from build123d import *

# Parameters (mm, degrees)
SKETCH_1_W          = 60
SKETCH_1_H          = 18
SKETCH_1_W_2        = 22.5
SKETCH_1_H_2        = 12
EXTRUDE_1_DEPTH     = 21
SKETCH_2_W          = 60
SKETCH_2_H          = 18
EXTRUDE_2_DEPTH     = 3
SKETCH_3_W          = 6
SKETCH_3_H          = 3
CUT_EXTRUDE_1_DEPTH = 6
SKETCH_4_R          = 2.75
EXTRUDE_3_DEPTH     = 5
SKETCH_6_R          = 1
CUT_EXTRUDE_2_DEPTH = 5
FILLET_1_R          = 1


with BuildPart() as part:
    # 草图1 → 凸台-拉伸1 (new body)
    with BuildSketch(Plane(origin=(0, 0, 0), x_dir=(1, 0, 0), z_dir=(0, 1, 0))):
        Rectangle(SKETCH_1_W, SKETCH_1_H)
        with Locations((-12.75, 0)):
            Rectangle(SKETCH_1_W_2, SKETCH_1_H_2, mode=Mode.SUBTRACT)
    extrude(amount=EXTRUDE_1_DEPTH)

    # 草图2 → 凸台-拉伸2 (add)
    with BuildSketch(Plane.XZ):
        Rectangle(SKETCH_2_W, SKETCH_2_H)
    extrude(amount=EXTRUDE_2_DEPTH)

    # 草图3 → 切除-拉伸1 (cut)
    with BuildSketch(Plane.ZY.offset(30)):
        with Locations((0, 1.5)):
            Rectangle(SKETCH_3_W, SKETCH_3_H)
    extrude(amount=-CUT_EXTRUDE_1_DEPTH, mode=Mode.SUBTRACT)

    # 草图4 → 凸台-拉伸3 (add)
    with BuildSketch(Plane.XZ.offset(3)):
        with Locations(Location((-18, 0, 0), (0, 0, 270))):
            Circle(SKETCH_4_R)
    extrude(amount=EXTRUDE_3_DEPTH)

    # 草图6 → 切除-拉伸2 (cut)
    with BuildSketch(Plane(origin=(0, 21, 0), x_dir=(1, 0, 0), z_dir=(0, 1, 0))):
        with Locations(Location((-26.75, 0, 0), (0, 0, 270))):
            Circle(SKETCH_6_R)
        with Locations(Location((1.25, 0, 0), (0, 0, 270))):
            Circle(SKETCH_6_R)
    extrude(amount=-CUT_EXTRUDE_2_DEPTH, mode=Mode.SUBTRACT)

    # 圆角1
    fillet_1_edges = [part.edges().sort_by_distance(p)[0] for p in [
        (-30, 21, 0),
        (0, 21, 9),
        (-30, -3, 0),
        (0, -3, -9),
        (30, -3, 0),
        (0, -3, 9),
        (30, 21, 0),
        (-30, 1.5, -3),
        (-30, 0, 0),
        (-30, 1.5, 3),
        (-30, 3, 0),
        (-18, -3, 2.75),
        (0, 21, -9),
        (30, 9, 9),
        (-30, 9, 9),
        (-30, 9, -9),
        (30, 9, -9),
    ]]
    fillet(fillet_1_edges, radius=FILLET_1_R)


solid = part.part
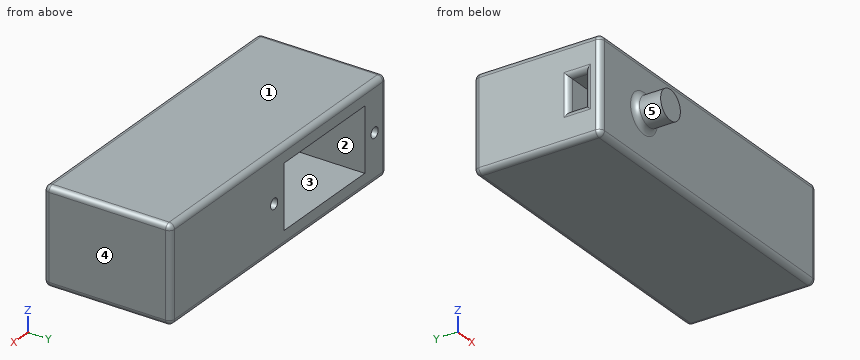
Part model, mm, in its own coordinate system. Face numbers are marked on the shaded views. A direction names the side the tool comes from. Coordinates: 2 decimals unless noted, no trailing zeros. Order: outer loops, then holes, each group sorted by start corner. A loop starts at its lowest first (then second) coordinate and runs counter-clockwise, first axis right, second up. Notation, with made-up numbers: M 44,21 L 77,21 A11 ccw 77,31 Z; hole C 70.25,41 d10. An arc over 180 degrees is marked long. One line per question, with ' | ' between items.
Q1. Slice it at D-D (x = 1.25). Give the cut face in (y, z), and give its area (3 significant figures).
A:
outline: M -3,-8 A1 ccw -2,-9 L 20,-9 A1 ccw 21,-8 L 21,-1 L 16,-1 L 16,1 L 21,1 L 21,8 A1 ccw 20,9 L -2,9 A1 ccw -3,8 Z | area: 421 mm^2
Q2. Drill centre lines: line 1 (X direction, y = 19.85, z = 0); line 2 (X direction, y = 17, z = 4.25); line 3 (Z direction, x = -2.5, y = 11.5). Where is each one in solid material? Low to high.
A:
line 1: x = -30 to -27.75, -25.75 to -24, -1.5 to 0.25, 2.25 to 30 | line 2: x = -30 to -24, -1.5 to 30 | line 3: z = -9 to -6, 6 to 9
Q3. Pin check, flat tips, straight feed: P1, Ø1.6, axis at x = 1, z = -0.5, coming from the +Y side; P2, Ø3.5, axis at x = -16, z = 0.5, coming from the +Y side; P3, Ø1.5, axis at x = -27, z = 0.5, coming from the -Y side; P4, Ø1.6, axis at x = 1.25, z = 0, coming from the +Y side. Stop position of each tip, or through.
A:
P1: stops at y = 21 | P2: stops at y = 0 | P3: stops at y = -3 | P4: stops at y = 16
Q4. 3-axis set-ups, long thin cutter, end or side, ignore diameter. For the marked faces 1 and 2: which of +Z, -Z, +X, -X, +Y, -Y reach the whole face in a straight line?
A:
face 1: +Z, +X, -X, +Y, -Y | face 2: +Y
Q5. Two-plate mould, pull along Z, no slides. Class the marked faces 3, 4 and 5: +Z half, -Z half, draft (parallel to the pull), parting line (faces both ways), or undercut.
A:
face 3: undercut | face 4: draft | face 5: parting line
Q6. Slice it at B-B (y = 19). Give the cut face in (x, z).
A:
outline: M -30,-8 A1 ccw -29,-9 L 29,-9 A1 ccw 30,-8 L 30,8 A1 ccw 29,9 L -29,9 A1 ccw -30,8 Z; hole C -26.75,0 d2; hole M -24,-6 L -1.5,-6 L -1.5,6 L -24,6 Z; hole C 1.25,0 d2
Q7. Slice it at C-C (x = -26.75). Give the cut face in (y, z).
A:
outline: M -3,-8 A1 ccw -2,-9 L 20,-9 A1 ccw 21,-8 L 21,-1 L 16,-1 L 16,1 L 21,1 L 21,8 A1 ccw 20,9 L -2,9 A1 ccw -3,8 Z; hole M 0,-3 L 3,-3 L 3,3 L 0,3 Z
